Work out the finished part from the listing and answer in its coordinate system (mm). Face numbers are marked on the shaded views. A direction names the side the tool comes from. Give positions to 0.01 mm unless a question says otherwise; leave off trailing zeros. Order: outer loops, then holes, each group sorted by start corner. A loop starts at its lowest first (then second) coordinate and runs counter-clockwise, first axis right, second up. Notation, with made-up numbers: (9.5, 44.5) - (44.5, 44.5) arc R16 cw to (44.5, 70.5) - close; hole circle Ø2 at (71.5, 21). An arc over 180 degrees is marked (long way). Return JSON: item names as keys, results as strings. Group by question number.
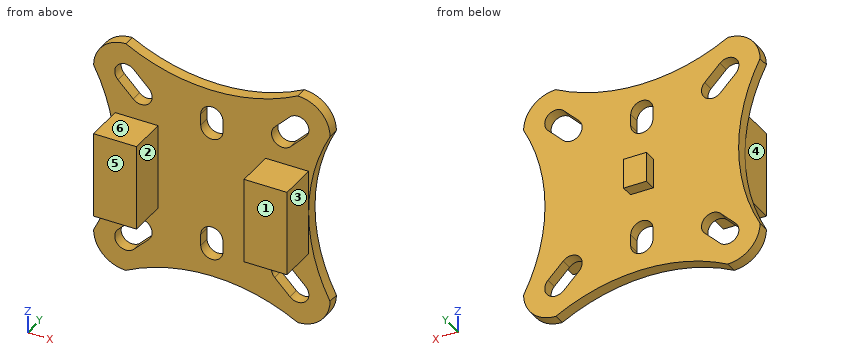
from build123d import *

# Parameters (mm, degrees)
BOSS_EXTRUDE1_DEPTH = 1.6
SKETCH2_W           = 3.2
SKETCH2_H           = 4.2
BOSS_EXTRUDE2_DEPTH = 1.7
SKETCH3_W           = 6
SKETCH3_H           = 12
BOSS_EXTRUDE3_DEPTH = 5.4


with BuildPart() as part:
    # Sketch1 → Boss-Extrude1 (new body)
    with BuildSketch(Plane(origin=(0, 0, 0), x_dir=(1, 0, 0), z_dir=(0, 1, 0))):
        with BuildLine():
            ThreePointArc((0, 4.5), (1.318019485, 1.318019485), (4.5, 0))
            ThreePointArc((4.5, 0), (16.5, 2.98672956), (28.5, 0))
            ThreePointArc((28.5, 0), (31.681980515, 1.318019485), (33, 4.5))
            ThreePointArc((33, 4.5), (30.01327044, 16.5), (33, 28.5))
            ThreePointArc((33, 28.5), (31.681980515, 31.681980515), (28.5, 33))
            ThreePointArc((28.5, 33), (16.5, 30.01327044), (4.5, 33))
            ThreePointArc((4.5, 33), (1.318019485, 31.681980515), (0, 28.5))
            ThreePointArc((0, 28.5), (2.98672956, 16.5), (0, 4.5))
        make_face()
        with BuildLine():
            Line((18.05, 26.05), (18.05, 24.45))
            ThreePointArc((18.05, 24.45), (16.5, 22.9), (14.95, 24.45))
            Line((14.95, 24.45), (14.95, 26.05))
            ThreePointArc((14.95, 26.05), (16.5, 27.6), (18.05, 26.05))
        make_face(mode=Mode.SUBTRACT)
        with BuildLine():
            Line((3.403984489, 5.596015511), (5.525304833, 7.717335854))
            ThreePointArc((5.525304833, 7.717335854), (7.717335854, 7.717335854), (7.717335854, 5.525304833))
            Line((7.717335854, 5.525304833), (5.596015511, 3.403984489))
            ThreePointArc((5.596015511, 3.403984489), (3.403984489, 3.403984489), (3.403984489, 5.596015511))
        make_face(mode=Mode.SUBTRACT)
        with BuildLine():
            Line((29.596015511, 5.596015511), (27.474695167, 7.717335854))
            ThreePointArc((27.474695167, 7.717335854), (25.282664146, 7.717335854), (25.282664146, 5.525304833))
            Line((25.282664146, 5.525304833), (27.403984489, 3.403984489))
            ThreePointArc((27.403984489, 3.403984489), (29.596015511, 3.403984489), (29.596015511, 5.596015511))
        make_face(mode=Mode.SUBTRACT)
        with BuildLine():
            Line((18.05, 6.95), (18.05, 8.55))
            ThreePointArc((18.05, 8.55), (16.5, 10.1), (14.95, 8.55))
            Line((14.95, 8.55), (14.95, 6.95))
            ThreePointArc((14.95, 6.95), (16.5, 5.4), (18.05, 6.95))
        make_face(mode=Mode.SUBTRACT)
        with BuildLine():
            Line((5.596015511, 29.596015511), (7.717335854, 27.474695167))
            ThreePointArc((7.717335854, 27.474695167), (7.717335854, 25.282664146), (5.525304833, 25.282664146))
            Line((5.525304833, 25.282664146), (3.403984489, 27.403984489))
            ThreePointArc((3.403984489, 27.403984489), (3.403984489, 29.596015511), (5.596015511, 29.596015511))
        make_face(mode=Mode.SUBTRACT)
        with BuildLine():
            Line((25.282664146, 27.474695167), (27.403984489, 29.596015511))
            ThreePointArc((27.403984489, 29.596015511), (29.596015511, 29.596015511), (29.596015511, 27.403984489))
            Line((29.596015511, 27.403984489), (27.474695167, 25.282664146))
            ThreePointArc((27.474695167, 25.282664146), (25.282664146, 25.282664146), (25.282664146, 27.474695167))
        make_face(mode=Mode.SUBTRACT)
    extrude(amount=BOSS_EXTRUDE1_DEPTH)

    # Sketch2 → Boss-Extrude2 (add)
    with BuildSketch(Plane(origin=(0, 1.6, 0), x_dir=(1, 0, 0), z_dir=(0, 1, 0))):
        with Locations((16.5, 16.5)):
            Rectangle(SKETCH2_W, SKETCH2_H)
    extrude(amount=BOSS_EXTRUDE2_DEPTH)

    # Sketch3 → Boss-Extrude3 (add)
    with BuildSketch(Plane.XZ):
        with Locations((6, -16.5)):
            Rectangle(SKETCH3_W, SKETCH3_H)
        with Locations((27, -16.5)):
            Rectangle(SKETCH3_W, SKETCH3_H)
    extrude(amount=BOSS_EXTRUDE3_DEPTH)


solid = part.part
1. The part is cut by section C-C (y = -2.75). Give the vertices of the cut face in (x, z), and give its area (3 significant figures).
2. Determine the mould class of the marked faces 1, 2 and 3 for opening direction X: released by +X, released by -X, zero draft, split by the parting line, or undercut.
3. The part is cut by section D-D (z = -27). Give the vertices of the cut face in (x, y).
4. A tool of negligible diameter and unlimited length cuts with its end or side. For the marked faces 4, 5 and 6, from which of +Z, -Z, +X, -X, +Y, -Y can it reach the whole face along a straight path? Write none if from no direction.
5. Consider probe 1 along X at (y, z) = (1, -29.5); probe 2 along X at (y, z) = (0.75, -28.5); probe 3 along X at (y, z) = (-4.25, -14.5). Determine where each line is inside the solid, lowest interval first. Write a range as from..to.
6. The part is cut by section A-A (y = 0.5). State how many separate pieces and enclosed holes the cut face has, and give its area (3 significant figures).
7. The part is cut by section B-B (x = 16.5). Give the vertices of the cut face in (y, z).
8. Each of these flat-tipped pins is pushed along its axis until it touches: pin 1 (1.9 mm diameter, centred on x = 16.5, y = 2, fed in from -Z); pin 2 (4.5 mm diameter, centred on x = 26.5, y = -3.5, fed in from +Z); pin 3 (1.6 mm diameter, centred on x = 5.5, y = -3, fed in from -Z). Where does it stop, or does it pass through?
Answers:
{
 "1": {"outline": "(3, -22.5) - (9, -22.5) - (9, -10.5) - (3, -10.5) - close; (24, -22.5) - (30, -22.5) - (30, -10.5) - (24, -10.5) - close", "area": "144 mm^2"},
 "2": {"face 1": "zero draft", "face 2": "undercut", "face 3": "released by +X"},
 "3": {"outline": "(0.73, 0) - (3.81, 0) - (3.81, 1.6) - (0.73, 1.6) - close; (8.04, 0) - (15.28, 0) - (15.28, 1.6) - (8.04, 1.6) - close; (17.72, 0) - (24.96, 0) - (24.96, 1.6) - (17.72, 1.6) - close; (29.19, 0) - (32.27, 0) - (32.27, 1.6) - (29.19, 1.6) - close"},
 "4": {"face 4": "+Z, -Z, -X, -Y", "face 5": "+Z, -Z, +X, -X, -Y", "face 6": "+Z, +X, -X, -Y"},
 "5": {"probe 1": "x = 0.11..3.32, 5.69..27.31, 29.68..32.89", "probe 2": "x = 0..2.95, 6.69..26.31, 30.05..33", "probe 3": "x = 3..9, 24..30"},
 "6": {"separate pieces": "1", "enclosed holes": "6", "area": "786 mm^2"},
 "7": {"outline": "(0, -30.01) - (1.6, -30.01) - (1.6, -27.6) - (0, -27.6) - close; (0, -22.9) - (1.6, -22.9) - (1.6, -18.6) - (3.3, -18.6) - (3.3, -14.4) - (1.6, -14.4) - (1.6, -10.1) - (0, -10.1) - close; (0, -5.4) - (1.6, -5.4) - (1.6, -2.99) - (0, -2.99) - close"},
 "8": {"pin 1": "stops at z = -30.03", "pin 2": "stops at z = -10.5", "pin 3": "stops at z = -22.5"}
}
